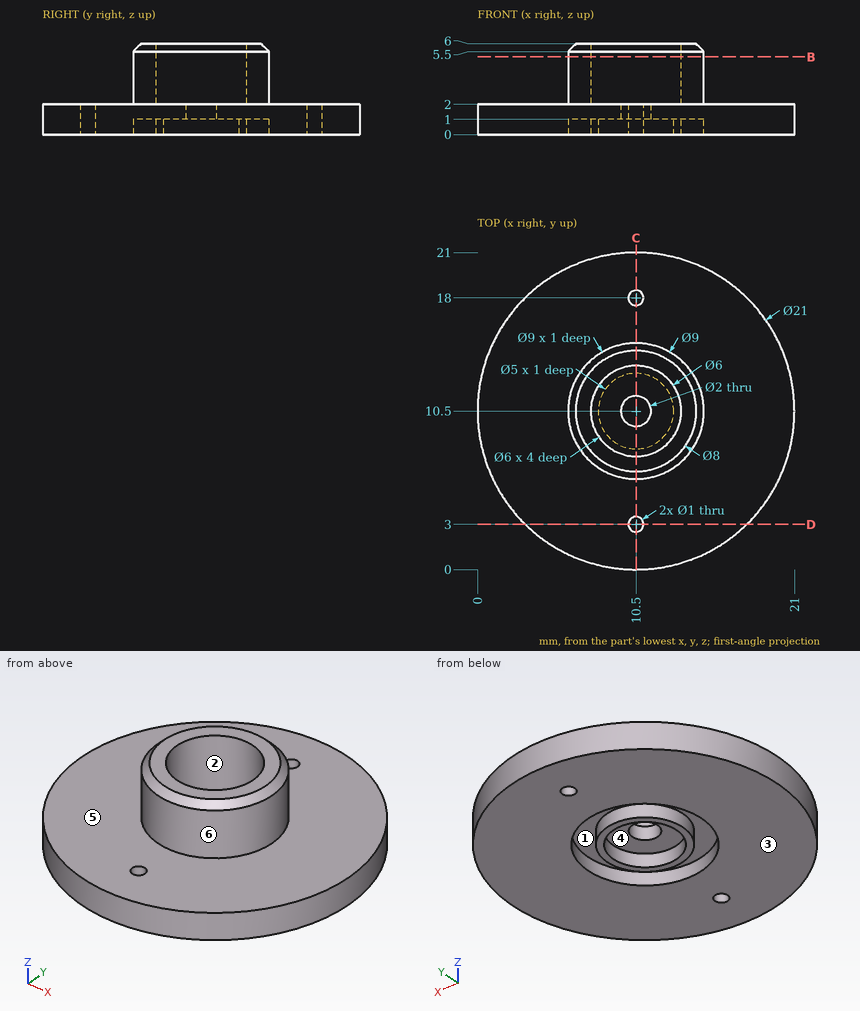
Part print with two shaded views. Sizes in mm from the minimum x, y, z corner. A direction names the side the tool comes from. Round coordinates to 2 decimals unless told otherwise and drop trailing zeros. Order: outer loops, then holes, each group sorted by start corner. A loop starts at its lowest first (then second) coordinate and runs counter-clockwise, first axis right, second up.
(1) 3-axis set-ups, long thin cutter, end or side, ignore diameter. For the marked faces 1, 2 and 3: which of +Z, -Z, +X, -X, +Y, -Y reach the whole face in a straight line?
(2) Pin check, flat tips, straight feed: pin 1 (1.5 mm diameter, centred on x = 2.5, y = 16.5, fed in from +Z); pin 2 (3 mm diameter, centred on x = 10.5, y = 10.5, fed in from -Z); pin 3 (3 mm diameter, centred on y = 7.5, z = 3, fed in from +X). Stop position of each tip, or through.
(3) Band-saw the part on B-B (z = 5.15). List the corners of the cut face in (x, y), then the cut area to 3 significant figures.
(4) Band-saw the part on C-C (x = 10.5). Give the number of separate pieces and of enclosed holes in the cut face, then the cut area to 4 significant figures.
(5) Pull direction X, two halves, no side cores. Call the marked faces 4, 5 and 6: released by +X, released by -X, zero draft, split by the parting line, or undercut.
(6) Drill centre lines: line 1 (Y direction, x = 10.5, z = 1.2); line 2 (Z direction, x = 6, y = 1.5); line 3 (Y direction, x = 8.25, z = 3.9). Where is each one in solid material? Low to high.
(7) Band-saw the part on D-D (y = 3). List the corners of the cut face in (x, z), then the cut area to 3 significant figures.
Verdict:
1. face 1: -Z
1. face 2: +Z
1. face 3: -Z, +X, -X, +Y, -Y
2. pin 1: stops at z = 2
2. pin 2: stops at z = 1
2. pin 3: stops at x = 20.83
3. outline: circle Ø9 at (10.5, 10.5); hole circle Ø6 at (10.5, 10.5)
3. area: 35.3 mm2
4. separate pieces: 4
4. enclosed holes: 0
4. area: 39.75 mm2
5. face 4: undercut
5. face 5: zero draft
5. face 6: split by the parting line
6. line 1: y = 0 to 2.5, 3.5 to 9.5, 11.5 to 17.5, 18.5 to 21
6. line 2: z = 0 to 2
6. line 3: y = 6.6 to 8.52, 12.48 to 14.4
7. outline: (3.15, 0) - (10, 0) - (10, 2) - (3.15, 2) - close; (11, 0) - (17.85, 0) - (17.85, 2) - (11, 2) - close
7. area: 27.4 mm2
